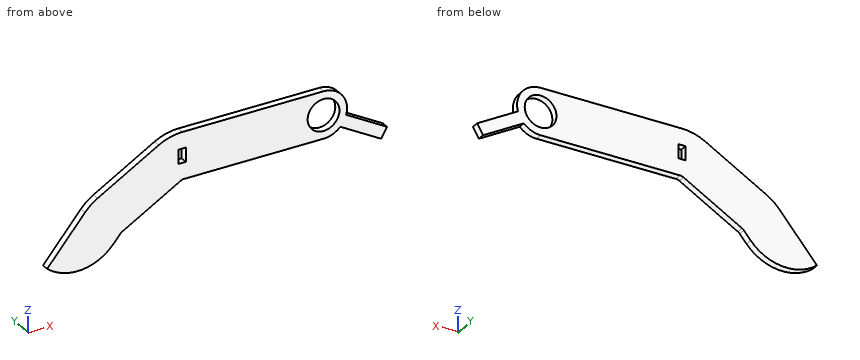
from build123d import *

# Parameters (mm, degrees)
F0_W     = 3
F0_H     = 6
F0_R     = 6.75
F1_DEPTH = 3
F2_R     = 3


with BuildPart() as f1:
    # F0 (on Front) → F1 (new body)
    with BuildSketch(Plane.XZ):
        with BuildLine():
            Line((-30, -10), (30, -10))
            ThreePointArc((30, -10), (33.868919, -9.221251), (37.135255, -7.006293))
            Line((37.135255, -7.006293), (54.455763, -17.006293))
            Line((54.455763, -17.006293), (56.955763, -12.676166))
            Line((56.955763, -12.676166), (39.635255, -2.676166))
            ThreePointArc((39.635255, -2.676166), (37.961208, 6.051378), (30, 10))
            Line((30, 10), (-30, 10))
            ThreePointArc((-30, 10), (-35.176381, 9.318517), (-40, 7.320508))
            Line((-40, 7.320508), (-65.980762, -7.679492))
            ThreePointArc((-65.980762, -7.679492), (-68.836514, -9.679111), (-71.301651, -12.144248))
            Line((-71.301651, -12.144248), (-87.371341, -31.295359))
            ThreePointArc((-87.371341, -31.295359), (-72.772474, -35.898364), (-59.1947, -28.830222))
            Line((-59.1947, -28.830222), (-55.980762, -25))
            Line((-55.980762, -25), (-30, -10))
        make_face()
        with Locations((-30, 0)):
            Rectangle(F0_W, F0_H, mode=Mode.SUBTRACT)
        with Locations((30, 0)):
            Circle(F0_R, mode=Mode.SUBTRACT)
    extrude(amount=F1_DEPTH)

    # F2
    f2_edges = [f1.edges().sort_by_distance(p)[0] for p in [
        (-30, -1.5, -10),
        (-55.980762, -1.5, -25),
    ]]
    fillet(f2_edges, radius=F2_R)


solid = f1.part
Part model, mm, in its own coordinate system. Coordinates: 2 decimals unless noted, no trailing zeros. Order: outer loops, then holes, each group sorted by start corner. A loop starts at its lowest first (then second) coordinate and runs counter-clockwise, first axis right, second up. Notation, with made-up numbers: M -29,-18 L -3,-18 A23 ccw -3,-10 Z; hole C -23,4.25 d6. An arc over 180 degrees is marked long. One line per question, with ' | ' between items.
Q1. Drill centre lines: line 1 (X direction, y = -0.2, z = -2); line 2 (Z direction, x = 30, y = -1.2); line 3 (Z direction, x = -20, y = -1.35). Where is each one in solid material? Low to high.
A:
line 1: x = -56.14 to -31.5, -28.5 to 23.55, 36.45 to 39.8 | line 2: z = -10 to -6.75, 6.75 to 10 | line 3: z = -10 to 10
Q2. Pin check, flat tips, straight feed: P1, Ø1.5, axis at y = -1.5, z = 0, coming from the +X side; P2, Ø0.9, axis at y = -1.5, z = -0.5, coming from the -X side; P3, Ø8, axis at x = -51, z = -25, coming from the -Y side; P4, Ø1.5, axis at y = -2, z = -9.5, coming from the +X side. Stop position of each tip, or through.
A:
P1: stops at x = 40 | P2: stops at x = -54.32 | P3: stops at y = -3 | P4: stops at x = 52.75
Q3. Slice it at A-A (y = -2.3). Give the cut face in (x, z).
A:
outline: M -87.37,-31.3 A20 ccw -59.19,-28.83 L -56.32,-25.41 A3 cw -55.52,-24.74 L -30.7,-10.4 A3 cw -29.2,-10 L 30,-10 A10 ccw 37.14,-7.01 L 54.46,-17.01 L 56.96,-12.68 L 39.64,-2.68 A10 ccw 30,10 L -30,10 A20 ccw -40,7.32 L -65.98,-7.68 A20 ccw -71.3,-12.14 Z; hole M -31.5,-3 L -28.5,-3 L -28.5,3 L -31.5,3 Z; hole C 30,0 d13.5
Q4. Slice it at D-D (x = -8.5). Give the cut face in (y, z), and give its area (3 significant figures).
A:
outline: M -3,-10 L 0,-10 L 0,10 L -3,10 Z | area: 60.0 mm^2
Q5. Slice it at C-C (z = -15.5). Give the cut face in (x, y).
A:
outline: M -74.12,-3 L -39.53,-3 L -39.53,0 L -74.12,0 Z; M 51.85,-3 L 55.33,-3 L 55.33,0 L 51.85,0 Z
Q6. Slice it at B-B (z = 0). Give the cut face in (x, y).
A:
outline: M -52.68,-3 L -31.5,-3 L -31.5,0 L -52.68,0 Z; M -28.5,-3 L 23.25,-3 L 23.25,0 L -28.5,0 Z; M 36.75,-3 L 40,-3 L 40,0 L 36.75,0 Z
